```python
from build123d import *

# Parameters (mm, degrees)
EXTRUDE_1_DEPTH     = 3
SKETCH_3_W          = 19
SKETCH_3_H          = 22
SKETCH_3_H_2        = 19
CUT_EXTRUDE_1_DEPTH = 3
FILLET_1_R          = 1
FILLET_2_R          = 2
FILLET_3_R          = 3
SKETCH_4_R          = 2.025
CUT_EXTRUDE_2_DEPTH = 3
SKETCH_5_R          = 2.025
CUT_EXTRUDE_3_DEPTH = 10


with BuildPart() as part:
    # 草图1 → 凸台-拉伸1 (new body)
    with BuildSketch(Plane.XY):
        Polygon((0, 0), (-70, 0), (-70, 20), (-55, 90), (-15, 90), (0, 20), align=None)
    extrude(amount=EXTRUDE_1_DEPTH)

    # 草图3 → 切除-拉伸1 (cut)
    with BuildSketch(Plane.XY.offset(3)):
        with Locations((-35, 67)):
            Rectangle(SKETCH_3_W, SKETCH_3_H)
        with Locations((-35, 37.5)):
            Rectangle(SKETCH_3_W, SKETCH_3_H_2)
        Polygon((-55, 70.909571916), (-55, 20), (-65.909193982, 20), align=None)
        Polygon((-4.090806018, 20), (-15, 70.909571916), (-15, 20), align=None)
    extrude(amount=-CUT_EXTRUDE_1_DEPTH, mode=Mode.SUBTRACT)

    # 圆角1
    fillet_1_edges = [part.edges().sort_by_distance(p)[0] for p in [
        (-4.090806018, 20, 1.5),
        (-15, 20, 1.5),
        (-15, 70.909571916, 1.5),
        (-65.909193982, 20, 1.5),
        (-55, 70.909571916, 1.5),
        (-55, 20, 1.5),
    ]]
    fillet(fillet_1_edges, radius=FILLET_1_R)

    # 圆角2
    fillet_2_edges = [part.edges().sort_by_distance(p)[0] for p in [
        (-25.5, 47, 1.5),
        (-25.5, 28, 1.5),
        (-44.5, 28, 1.5),
        (-44.5, 47, 1.5),
        (-25.5, 78, 1.5),
        (-25.5, 56, 1.5),
        (-44.5, 56, 1.5),
        (-44.5, 78, 1.5),
    ]]
    fillet(fillet_2_edges, radius=FILLET_2_R)

    # 圆角3
    fillet_3_edges = [part.edges().sort_by_distance(p)[0] for p in [
        (0, 0, 1.5),
        (-70, 0, 1.5),
        (-70, 20, 1.5),
        (-55, 90, 1.5),
        (-15, 90, 1.5),
        (0, 20, 1.5),
    ]]
    fillet(fillet_3_edges, radius=FILLET_3_R)

    # 草图4 → 切除-拉伸2 (cut)
    with BuildSketch(Plane.XY.offset(3)):
        with Locations((-62.5, 10)):
            Circle(SKETCH_4_R)
        with Locations((-35, 10)):
            Circle(SKETCH_4_R)
        with Locations((-7.5, 10)):
            Circle(SKETCH_4_R)
    extrude(amount=-CUT_EXTRUDE_2_DEPTH, mode=Mode.SUBTRACT)

    # 草图5 → 切除-拉伸3 (cut)
    with BuildSketch(Plane(origin=(0, 0, 0), x_dir=(-1, 0, 0), z_dir=(0, 0, -1))):
        with Locations((35, 82.566965626)):
            Circle(SKETCH_5_R)
        with Locations((35, 51.566965626)):
            Circle(SKETCH_5_R)
        with Locations((35, 24)):
            Circle(SKETCH_5_R)
    extrude(amount=-CUT_EXTRUDE_3_DEPTH, mode=Mode.SUBTRACT)


solid = part.part
```
The model under review builds one solid part; all positions refer to its coordinate system, in mm. A direction names the side the tool comes from. Give positions to 0.01 mm unless a question says otherwise; leave off trailing zeros. Order: outer loops, then holes, each group sorted by start corner. A loop starts at its lowest first (then second) coordinate and runs counter-clockwise, first axis right, second up. Notation, with made-up numbers: (-38.75, 74.25) - (9.25, 74.25) arc R16 ccw to (9.25, 98.25) - close; hole circle Ø2 at (81.5, 30). An arc over 180 degrees is marked (long way). Use CSV: the item, a comma, the result in double quotes. Start each with the question number.
Q1. We need section A-A, the plane x = -28.5. Write out the cut boundary in (y, z).
Q2. We need section C-C, the plane y = 69. Write out the cut boundary in (x, z).
Q3. We need section D-D, the plane x = -43.5. Write out the cut boundary in (y, z).
Q4. Tool access review of faces 1 (the cylindrical face through (-26.07, 28.6, 1.48)), 2 (the cylindrical face through (-15.5, 89.3, 1.5)): name each direction out of +Z, -Z, +X, -X, +Y, -Y from which nothing blocks a thin tool from reaching the whole face with its end or side.
Q5. We need section B-B, the plane y = 10. Write out the cut boundary in (x, z) (3 decimals).
Q6. To check wall thickness, follow line 1 along Y through (x, z) = (-29, 2.05); line 2 along X through (y, z) = (31, 0.75); line 3 along X through (y, z) = (42, 2.2). State the ranges of each line that lie inside material, in increasing order. Write a range as [from, to].
Q7. Clearance check with flat-ended pins moving along their axes: pin 1 Ø2.5 at (x, y) = (-35, 10) entering from -Z; pin 2 Ø1.5 at (y, z) = (37.5, 2) entering from +X. State where each tip first meets the part, or that it passes through.
Q8. The part is to be moulded in two halves that separate along Y. For faces 3 (the flat face through (-70, 11, 1)), 4 (the cylindrical face through (-60.63, 9.22, 1.52)), 5 (the flat face through (-7.38, 54.44, 1.48)), 6 (the cylindrical face through (-14.13, 62.46, 1.48)), say which applies: +Y half, -Y half, draft (parallel to the pull), parting line (faces both ways), or undercut.
Outcome:
1,outline,"(0, 0) - (28, 0) - (28, 3) - (0, 3) - close; (47, 0) - (56, 0) - (56, 3) - (47, 3) - close; (78, 0) - (90, 0) - (90, 3) - (78, 3) - close"
2,outline,"(-59.5, 0) - (-44.5, 0) - (-44.5, 3) - (-59.5, 3) - close; (-25.5, 0) - (-10.5, 0) - (-10.5, 3) - (-25.5, 3) - close"
3,outline,"(0, 0) - (28.27, 0) - (28.27, 3) - (0, 3) - close; (46.73, 0) - (56.27, 0) - (56.27, 3) - (46.73, 3) - close; (77.73, 0) - (90, 0) - (90, 3) - (77.73, 3) - close"
4,face 1,"+Z, -Z"
4,face 2,"+Z, -Z, +X, +Y"
5,outline,"(-70, 0) - (-64.525, 0) - (-64.525, 3) - (-70, 3) - close; (-60.475, 0) - (-37.025, 0) - (-37.025, 3) - (-60.475, 3) - close; (-32.975, 0) - (-9.525, 0) - (-9.525, 3) - (-32.975, 3) - close; (-5.475, 0) - (0, 0) - (0, 3) - (-5.475, 3) - close"
6,line 1,"y = [0, 28], [47, 56], [78, 90]"
6,line 2,"x = [-67.64, -63.55], [-55, -44.5], [-25.5, -15], [-6.45, -2.36]"
6,line 3,"x = [-65.29, -61.19], [-55, -44.5], [-25.5, -15], [-8.81, -4.71]"
7,pin 1,"passes through"
7,pin 2,"stops at x = -3.59"
8,face 3,"draft"
8,face 4,"undercut"
8,face 5,"+Y half"
8,face 6,"undercut"
